Input: dimensioned drawing with shaded views. Units: mm. Origin: part minimum x, y, z. A direction names the side the tool comes from. Round coordinates to 2 decimals unless told otherwise and drop trailing zeros. Write each loop counter-clockwise with the first axis right and the second up, starting at its lowest first coordinate (ties: lowest second). Pieces come first, ordered by that corner, then holes. Notation, with made-up numbers: (-11.75, 39.25) - (-1.75, 39.25) arc R9 ccw to (-1.75, 48.25) - close; hole circle Ø1 at (-10, 10). An arc over 180 degrees is marked (long way). Write item = value, one per line. Start each with the question number.
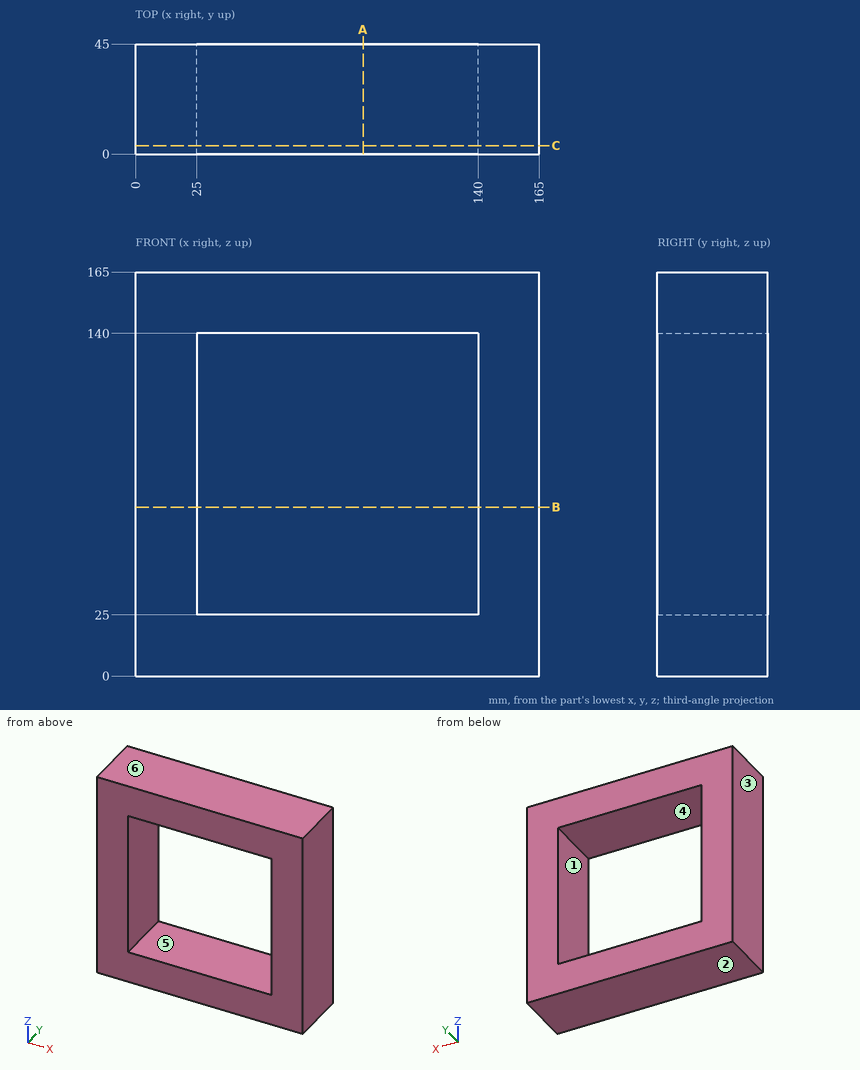
(1) Section C-C (y = 3.5). Return the cut outline in (x, z), plus the area to 3 significant figures.
(2) Reachability of the marked faces 5 and 6 from +Z, -Z, +X, -X, +Y, -Y: full face, straight path, thin tool, end or side. Return the list, or none.
(3) Ray query, L1, parallel to X at y = 23, z = 102. Return the intervals inside material, ascending. Write a range as from..to.
(4) Section A-A (x = 93). Return the cut outline in (y, z), plus the area to 3 significant figures.
(5) Section B-B (z = 69). Return the cut outline in (x, y), plus the area to 3 significant figures.
(6) Pull-direction query (Z, two-part tool) for the marked faces 1, 2, 3 and 4; classes: +Z half, -Z half, draft (parallel to the pull), parting line (faces both ways), or undercut.
(7) Contact query for a flat-ended pin moving along its axis: P1, Ø13.5, axis at x = 109, y = 28, coming from the -Z side. Output: stop coordinate, or through.
Solution:
q1.outline = (0, 0) - (165, 0) - (165, 165) - (0, 165) - close; hole (25, 25) - (140, 25) - (140, 140) - (25, 140) - close
q1.area = 14,000 mm^2
q2.face_5 = +Y, -Y
q2.face_6 = +Z, +X, -X, +Y, -Y
q3.L1 = 0..25, 140..165
q4.outline = (0, 0) - (45, 0) - (45, 25) - (0, 25) - close; (0, 140) - (45, 140) - (45, 165) - (0, 165) - close
q4.area = 2,250 mm^2
q5.outline = (0, 0) - (25, 0) - (25, 45) - (0, 45) - close; (140, 0) - (165, 0) - (165, 45) - (140, 45) - close
q5.area = 2,250 mm^2
q6.face_1 = undercut
q6.face_2 = -Z half
q6.face_3 = draft
q6.face_4 = undercut
q7.P1 = 0
